from build123d import *

# Parameters (mm, degrees)
SKETCH2_W          = 15.494
SKETCH2_H          = 15.494
CUT_EXTRUDE1_DEPTH = 12.7


with BuildPart() as part:
    # Sketch1 → Revolve1 (revolve)
    with BuildSketch(Plane.XY, mode=Mode.PRIVATE) as revolve1_sk:
        Polygon((165.1, 0), (165.1, 15.875), (0, 19.05), (0, 0), (12.7, 0), align=None)
    revolve(revolve1_sk.sketch.rotate(Axis((0, 19.05, 0), (0.9998151400298467, -0.01922721423134321, 0)), 180), axis=Axis((0, 19.05, 0), (0.9998151400298467, -0.01922721423134321, 0)))

    # Sketch2 → Cut-Extrude1 (cut, symmetric)
    with BuildSketch(Plane(origin=(165.1, 0, 0), x_dir=(0, 0, -1), z_dir=(1, 0, 0))):
        with Locations((0, 15.875)):
            Rectangle(SKETCH2_W, SKETCH2_H)
    extrude(amount=CUT_EXTRUDE1_DEPTH, both=True, mode=Mode.SUBTRACT)


solid = part.part
For this review, take the finished solid that the model builds, in its own axes (mm). A direction names the side the tool comes from. Round coordinates to 2 decimals unless told otherwise and drop trailing zeros. Answer as CSV lines item,"result".
(1) Mouldability with a two-part tool opening along Y and no side actions: class faces 4 (the face through (84.36, 34.06, 5.24)), 5 (the face through (159, 23.622, 0)) as +Y half, -Y half, draft (parallel to the pull), parting line (faces both ways), or undercut.
Checked values:
face 4,"parting line"
face 5,"undercut"
(2) Insertion check: P1, Ø2, axis at x = 141, y = 19.5, coming from the -Z side; P2, Ø4, axis at x = 22.5, z = 7.5, coming from the -Y side; P3, Ø8, axis at y = 27, z = 9.5, coming from the -X side; P4, Ø14.5, axis at x = 157.5, z = -1, coming from the -Y side. Each pin has a flat end and moves straight along its axis. Give the tip position at first contact, or say it passes through.
Checked values:
P1,"stops at z = -16.2"
P2,"stops at y = 0.83"
P3,"stops at x = 0.25"
P4,"stops at y = 0"
(3) Wall thickness on line 1 (X direction, y = 4, z = 6); line 2 (X direction, y = 16.5, z = -1); line 3 (Y direction, x = 32.5, z = 6): over which ranges is each line inside the solid? List them lowest first.
Checked values:
line 1,"x = 0.02 to 165.13"
line 2,"x = 0 to 152.4"
line 3,"y = 1 to 35.86"
(4) Tool access review of faces 1 (the face through (159, 16, 7.747)), 2 (the face through (0, 18, 0)), 3 (the face through (165.223, 14.108, -7.947)): name each direction out of +Z, -Z, +X, -X, +Y, -Y from which nothing blocks a thin tool from reaching the whole face with its end or side.
Checked values:
face 1,"+X"
face 2,"-X, +Y"
face 3,"+X, -Y"
